from build123d import *

# Parameters (mm, degrees)
BODYSCH_R  = 14.224
BODY_DEPTH = 23.876
FLOWSCH_R  = 8.5344
FLOW_DEPTH = 47.752
FILLET1_R  = 1.0668


with BuildPart() as part:
    # BodySch → Body (new, symmetric)
    with BuildSketch(Plane.XY):
        Circle(BODYSCH_R)
    extrude(amount=BODY_DEPTH, both=True)

    # FlowSch → Flow (cut)
    with BuildSketch(Plane.XY.offset(-23.876)):
        Circle(FLOWSCH_R)
    extrude(amount=FLOW_DEPTH, mode=Mode.SUBTRACT)

    # ThreadSch → Thread (revolve, cut)
    with BuildSketch(Plane(origin=(0, 0, 0), x_dir=(0, 0, -1), z_dir=(1, 0, 0)), mode=Mode.PRIVATE) as thread_sk:
        Polygon((-10.32002, 0), (-10.32002, 10.245933299), (-23.876, 10.668), (-23.876, 0), align=None)
    thread = revolve(thread_sk.sketch.rotate(Axis((0, 0, 0), (0, 0, 1)), 90), axis=Axis((0, 0, 0), (0, 0, 1)), mode=Mode.SUBTRACT)

    # Fillet1
    fillet1_edges = [part.edges().sort_by_distance(p)[0] for p in [
        (-14.224, 0, -23.876),
        (-14.224, 0, 23.876),
    ]]
    fillet(fillet1_edges, radius=FILLET1_R)

    # Mirror1: Thread across plane
    add(thread.mirror(Plane.XY), mode=Mode.SUBTRACT)


solid = part.part
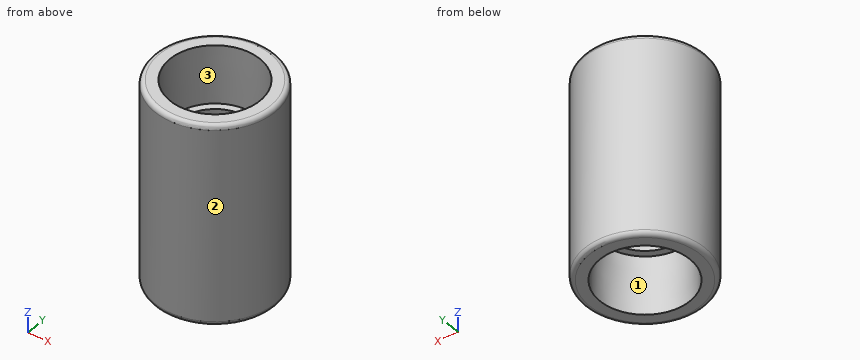
Build history of the part. All positions in model axes, mm. Face numbers are marked on the shaded views. Give positions to 0.01 mm unless a question says otherwise; leave off trailing zeros. Order: outer loops, then holes, each group sorted by start corner. A loop starts at its lowest first (then second) coordinate and runs counter-clockwise, first axis right, second up. Notation, with made-up numbers: M 39.25,86 L 73.25,86 A15 cw 73.25,101 Z; hole C 72.5,23 d2. An arc over 180 degrees is marked long. Use one line per item in the form item = value.
1) Saw through at A-A (y = 0). Give the cut face in (x, z), plus the area to 3 significant figures.
Calculated:
outline = M -14.22,-22.81 A1.07 ccw -13.16,-23.88 L -10.67,-23.88 L -10.25,-10.32 L -8.53,-10.32 L -8.53,10.32 L -10.25,10.32 L -10.67,23.88 L -13.16,23.88 A1.07 ccw -14.22,22.81 Z; M 8.53,-10.32 L 10.25,-10.32 L 10.67,-23.88 L 13.16,-23.88 A1.07 ccw 14.22,-22.81 L 14.22,22.81 A1.07 ccw 13.16,23.88 L 10.67,23.88 L 10.25,10.32 L 8.53,10.32 Z
area = 438 mm2
2) Drop flat-ended pins along their axis: pin 1 (1 mm diameter, centred on x = -4.5, z = -1.5, fed in from +Y); pin 2 (5 mm diameter, centred on y = 5.5, z = -19, fed in from -X); pin 3 (12 mm diameter, centred on y = 10, z = -1.5, fed in from +X). Give the stop position or say it passes through.
Calculated:
pin_1 = 13.65
pin_2 = -13.9
pin_3 = 13.65
3) Saw through at D-D (z = 14.5). Give the cut face in (x, y).
Calculated:
outline = C 0,0 d28.45; hole C 0,0 d20.75
4) Two-plate mould, pull along X, no slides. Class the marked faces 1, 2 and 3: released by +X, released by -X, zero draft, split by the parting line, or undercut.
Calculated:
face_1 = undercut
face_2 = split by the parting line
face_3 = undercut
5) Saw through at C-C (z = -7.5). Give the cut face in (x, y), plus the area to 3 significant figures.
Calculated:
outline = C 0,0 d28.45; hole C 0,0 d17.07
area = 407 mm2
6) Probe probe 1 along Y at (x, z) = (0, 2.5); probe 2 along X at (y, z) = (5, -18); probe 3 along X at (y, z) = (-8.5, 14). List the from-to ranges inside material, lowest first.
Calculated:
probe_1 = -14.22 to -8.53, 8.53 to 14.22
probe_2 = -13.32 to -9.22, 9.22 to 13.32
probe_3 = -11.4 to -5.92, 5.92 to 11.4
